```python
from build123d import *

# Parameters (mm, degrees)
BOSS_EXTRU_1_DEPTH = 23


with BuildPart() as part:
    # Esquisse1 → Boss.-Extru.1 (new body)
    with BuildSketch(Plane(origin=(0, 0, 0), x_dir=(1, 0, 0), z_dir=(0, 1, 0))):
        Polygon((7, 11), (8, 11), (8, 1), (12, 1), (12, 11), (13, 11), (13, -3.968463396), (13, -5), (12, -5), (12, 0), (-12, 0), (-12, -5), (-13, -5), (-13, -3.968463396), (-13, 11), (-12, 11), (-12, 1), (-8, 1), (-8, 11), (-7, 11), (-7, 1), (-3, 1), (-3, 11), (-2, 11), (-2, 1), (2, 1), (2, 11), (3, 11), (3, 1), (7, 1), align=None)
    extrude(amount=BOSS_EXTRU_1_DEPTH)


solid = part.part
```
Source: CAD feature listing. Evaluate the final solid. Frame: model axes, mm. A direction names the side the tool comes from. Give positions to 0.01 mm unless a question says otherwise; leave off trailing zeros. Loops run counter-clockwise (first coordinate to the right, second up) from the corner with the lowest first, then second, coordinate; pieces in that order, holes last. Notation, with made-up numbers: (5.25, 88) - (37.25, 88) arc R9 cw to (37.25, 96) - close; hole circle Ø10 at (53.5, -18). An arc over 180 degrees is marked (long way). Use CSV: the item, a comma, the result in double quotes.
1) Pin query (flat end, axial travel): P1, Ø11.5, axis at x = -4.5, y = 6, coming from the +Z side; P2, Ø1.2, axis at x = -5.5, y = 10, coming from the -Z side. Return the tip coordinate at first contact, or that it passes through.
Worked out:
P1,"stops at z = 0"
P2,"stops at z = -1"
2) Cut plane C-C (y = 16.5). Output: boundary loops of the cut face in (x, z), and give its area (3 significant figures).
Worked out:
outline,"(-13, -11) - (-12, -11) - (-12, -1) - (-8, -1) - (-8, -11) - (-7, -11) - (-7, -1) - (-3, -1) - (-3, -11) - (-2, -11) - (-2, -1) - (2, -1) - (2, -11) - (3, -11) - (3, -1) - (7, -1) - (7, -11) - (8, -11) - (8, -1) - (12, -1) - (12, -11) - (13, -11) - (13, 5) - (12, 5) - (12, 0) - (-12, 0) - (-12, 5) - (-13, 5) - close"
area,"96.0 mm^2"
3) Set-up query: faces 4 (the flat face through (0, 11, 0)), 5 (the flat face through (7.5, 11.3, -11)), 6 (the flat face through (-8, 11, -6)). Return all of +Z, -Z, +X, -X, +Y, -Y with unobstructed straight access to the full face (end or side cutting, diameter ignored); none if empty.
Worked out:
face 4,"+Z, +Y, -Y"
face 5,"-Z, +X, -X, +Y, -Y"
face 6,"-Z, +Y, -Y"
4) Cut plane B-B (z = 1.5). Output: boundary loops of the cut face in (x, y).
Worked out:
outline,"(-13, 0) - (-12, 0) - (-12, 23) - (-13, 23) - close; (12, 0) - (13, 0) - (13, 23) - (12, 23) - close"
5) Mould query, pull axis X, two halves, no side actions, for faces 1 (the flat face through (2.5, 11.3, -11)), 2 (the flat face through (12, 11, -6)), 3 (the flat face through (0, 11, -1)). Classes: +X half, -X half, draft (parallel to the pull), parting line (faces both ways), or undercut.
Worked out:
face 1,"draft"
face 2,"undercut"
face 3,"undercut"
6) Cut plane D-D (x = 2.5). Output: boundary loops of the cut face in (y, z), and give its area (3 significant figures).
Worked out:
outline,"(0, -11) - (23, -11) - (23, 0) - (0, 0) - close"
area,"253 mm^2"
7) Line query: line 1 (X direction, y = 3, z = -3); line 2 (X direction, y = 20, z = 2.25); line 3 (Z direction, x = 4.75, y = 13.5). Output: solid intervals per line, ascending.
Worked out:
line 1,"x = -13 to -12, -8 to -7, -3 to -2, 2 to 3, 7 to 8, 12 to 13"
line 2,"x = -13 to -12, 12 to 13"
line 3,"z = -1 to 0"
8) Cut plane A-A (z = -9.75). Output: boundary loops of the cut face in (x, y), and give its area (3 significant figures).
Worked out:
outline,"(-13, 0) - (-12, 0) - (-12, 23) - (-13, 23) - close; (-8, 0) - (-7, 0) - (-7, 23) - (-8, 23) - close; (-3, 0) - (-2, 0) - (-2, 23) - (-3, 23) - close; (2, 0) - (3, 0) - (3, 23) - (2, 23) - close; (7, 0) - (8, 0) - (8, 23) - (7, 23) - close; (12, 0) - (13, 0) - (13, 23) - (12, 23) - close"
area,"138 mm^2"
